from build123d import *

# Parameters (mm, degrees)
SKETCH2_W           = 115
SKETCH2_H           = 130
SKETCH2_R           = 4.8
BOSS_EXTRUDE1_DEPTH = 5
BOSS_EXTRUDE2_DEPTH = 115
SKETCH4_W           = 98.530736165
SKETCH4_H           = 115
CUT_EXTRUDE1_DEPTH  = 5
SKETCH5_R           = 4.8
CUT_EXTRUDE2_DEPTH  = 1
SKETCH6_R           = 4.8
CUT_EXTRUDE4_DEPTH  = 1
SKETCH7_W           = 19
SKETCH7_H           = 115
BOSS_EXTRUDE3_DEPTH = 39.811986363
SKETCH8_W           = 19
SKETCH8_H           = 115
SKETCH8_W_2         = 31.469263835
BOSS_EXTRUDE4_DEPTH = 100
CUT_EXTRUDE5_DEPTH  = 19
CUT_EXTRUDE6_DEPTH  = 31.469263835
CUT_EXTRUDE7_DEPTH  = 5
SKETCH12_W          = 5
SKETCH12_H          = 10
BOSS_EXTRUDE5_DEPTH = 100
CHAMFER1_SIZE       = 3
SKETCH13_W          = 5
SKETCH13_H          = 31
BOSS_EXTRUDE6_DEPTH = 5


with BuildPart() as part:
    # Sketch2 → Boss-Extrude1 (new body)
    with BuildSketch(Plane(origin=(0, 0, 0), x_dir=(0, 1, 0), z_dir=(0, 0, 1))):
        Rectangle(SKETCH2_W, SKETCH2_H)
        with Locations(Location((-18.09, -55.5, 0), (0, 0, 270))):
            Circle(SKETCH2_R, mode=Mode.SUBTRACT)
        with Locations(Location((18.08, -55.5, 0), (0, 0, 270))):
            Circle(SKETCH2_R, mode=Mode.SUBTRACT)
    extrude(amount=BOSS_EXTRUDE1_DEPTH)

    # Sketch3 → Boss-Extrude2 (add)
    with BuildSketch(Plane(origin=(0, 57.5, 0), x_dir=(-1, 0, 0), z_dir=(0, 1, 0))):
        Polygon((-65, 5), (-46, 5), (46, 45.27), (65, 45.27), (65, 39.811986363), (46, 39.811986363), (-33.530736165, 5), (-33.530736165, 0), (-65, 0), align=None)
    extrude(amount=-BOSS_EXTRUDE2_DEPTH)

    # Sketch4 → Cut-Extrude1 (cut)
    with BuildSketch(Plane.XY.offset(5)):
        with Locations((-15.734631917, 0)):
            Rectangle(SKETCH4_W, SKETCH4_H)
    extrude(amount=-CUT_EXTRUDE1_DEPTH, mode=Mode.SUBTRACT)

    # Sketch5 → Cut-Extrude2 (cut)
    with BuildSketch(Plane.XY.offset(5)):
        with Locations((56.5, 7.5)):
            Circle(SKETCH5_R)
        with Locations((56.5, -7.5)):
            Circle(SKETCH5_R)
    extrude(amount=-CUT_EXTRUDE2_DEPTH, mode=Mode.SUBTRACT)

    # Sketch6 → Cut-Extrude4 (cut)
    with BuildSketch(Plane.XY.offset(45.27)):
        with Locations((-55.5, 17.65)):
            Circle(SKETCH6_R)
        with Locations((-55.5, -17.65)):
            Circle(SKETCH6_R)
    extrude(amount=-CUT_EXTRUDE4_DEPTH, mode=Mode.SUBTRACT)

    # Sketch7 → Boss-Extrude3 (add)
    with BuildSketch(Plane(origin=(0, 0, 39.811986363), x_dir=(1, 0, 0), z_dir=(0, 0, -1))):
        with Locations((-55.5, 0)):
            Rectangle(SKETCH7_W, SKETCH7_H)
    extrude(amount=BOSS_EXTRUDE3_DEPTH)

    # Sketch8 → Boss-Extrude4 (add)
    with BuildSketch(Plane(origin=(0, 0, 0), x_dir=(1, 0, 0), z_dir=(0, 0, -1))):
        with Locations((-55.5, 0)):
            Rectangle(SKETCH8_W, SKETCH8_H)
        with Locations((49.265368083, 0)):
            Rectangle(SKETCH8_W_2, SKETCH8_H)
    extrude(amount=BOSS_EXTRUDE4_DEPTH)

    # Sketch9 → Cut-Extrude5 (cut)
    with BuildSketch(Plane(origin=(-65, 0, 0), x_dir=(0, -1, 0), z_dir=(-1, 0, 0))):
        with BuildLine():
            Line((-37.5, -95), (37.5, -95))
            ThreePointArc((37.5, -95), (44.571067812, -92.071067812), (47.5, -85))
            Line((47.5, -85), (47.5, 20.27))
            ThreePointArc((47.5, 20.27), (44.571067812, 27.341067812), (37.5, 30.27))
            Line((37.5, 30.27), (-37.5, 30.27))
            ThreePointArc((-37.5, 30.27), (-44.571067812, 27.341067812), (-47.5, 20.27))
            Line((-47.5, 20.27), (-47.5, -85))
            ThreePointArc((-47.5, -85), (-44.571067812, -92.071067812), (-37.5, -95))
        make_face()
    extrude(amount=-CUT_EXTRUDE5_DEPTH, mode=Mode.SUBTRACT)

    # Sketch10 → Cut-Extrude6 (cut)
    with BuildSketch(Plane.YZ.offset(65)):
        with BuildLine():
            Line((-40, -95), (40, -95))
            ThreePointArc((40, -95), (47.071067812, -92.071067812), (50, -85))
            Line((50, -85), (50, -15))
            ThreePointArc((50, -15), (47.071067812, -7.928932188), (40, -5))
            Line((40, -5), (-40, -5))
            ThreePointArc((-40, -5), (-47.071067812, -7.928932188), (-50, -15))
            Line((-50, -15), (-50, -85))
            ThreePointArc((-50, -85), (-47.071067812, -92.071067812), (-40, -95))
        make_face()
    extrude(amount=-CUT_EXTRUDE6_DEPTH, mode=Mode.SUBTRACT)

    # Sketch11 → Cut-Extrude7 (cut)
    with BuildSketch(Plane(origin=(9.233013436, 0, 21.093549445), x_dir=(0.9160841896254345, 0, -0.4009859816980028), z_dir=(0.4009859816980028, 0, 0.9160841896254345))):
        with BuildLine():
            Line((-40.292508114, 47.5), (20.134942814, 47.5))
            ThreePointArc((20.134942814, 47.5), (27.206010626, 44.571067812), (30.134942814, 37.5))
            Line((30.134942814, 37.5), (30.134942814, -37.5))
            ThreePointArc((30.134942814, -37.5), (27.206010626, -44.571067812), (20.134942814, -47.5))
            Line((20.134942814, -47.5), (-40.292508114, -47.5))
            ThreePointArc((-40.292508114, -47.5), (-47.363575926, -44.571067812), (-50.292508114, -37.5))
            Line((-50.292508114, -37.5), (-50.292508114, 37.5))
            ThreePointArc((-50.292508114, 37.5), (-47.363575926, 44.571067812), (-40.292508114, 47.5))
        make_face()
    extrude(amount=-CUT_EXTRUDE7_DEPTH, mode=Mode.SUBTRACT)

    # Sketch12 → Boss-Extrude5 (add)
    with BuildSketch(Plane.ZY.offset(65)):
        with Locations((-97.5, 52.5)):
            Rectangle(SKETCH12_W, SKETCH12_H)
        with Locations((-97.5, -52.5)):
            Rectangle(SKETCH12_W, SKETCH12_H)
    extrude(amount=-BOSS_EXTRUDE5_DEPTH)

    # Chamfer1
    chamfer1_edges = [part.edges().sort_by_distance(p)[0] for p in [
        (-46, 52.5, -95),
        (33.530736165, 52.5, -95),
        (-46, -52.5, -95),
        (33.530736165, -52.5, -95),
    ]]
    chamfer(chamfer1_edges, length=CHAMFER1_SIZE)

    # Sketch13 → Boss-Extrude6 (add)
    with BuildSketch(Plane(origin=(65, 0, 0), x_dir=(0, 0, -1), z_dir=(1, 0, 0))):
        with Locations((97.5, 42)):
            Rectangle(SKETCH13_W, SKETCH13_H)
    extrude(amount=BOSS_EXTRUDE6_DEPTH)


solid = part.part
Verification items for the finished model (mm, model axes). A direction names the side the tool comes from. Coordinates: 2 decimals unless noted, no trailing zeros. Write each loop counter-clockwise with the first axis right and the second up, starting at its lowest first coordinate (ties: lowest second). Pieces come first, ordered by that corner, then holes. Notation, with made-up numbers: M 45,-31 L 92,-31 A20 cw 92,-4 Z; hole C -19,73.25 d1. An arc over 180 degrees is marked long. Use CSV: the item, a comma, the result in double quotes.
Q1. Section check A-A, the plane z = -29. Enter the section's corners in (x, y), and give its area (3 significant figures).
Computed values:
outline,"M -65,-57.5 L -46,-57.5 L -46,-47.5 L -65,-47.5 Z; M -65,47.5 L -46,47.5 L -46,57.5 L -65,57.5 Z; M 33.53,-57.5 L 65,-57.5 L 65,-50 L 33.53,-50 Z; M 33.53,50 L 65,50 L 65,57.5 L 33.53,57.5 Z"
area,"852 mm²"
Q2. Go/stop test with flat-tipped pins: P1, Ø11, axis at x = 56.5, y = 7.5, coming from the +Z side; P2, Ø7.5, axis at x = -55.5, y = 17.65, coming from the +Z side; P3, Ø1, axis at x = 39, y = 32, coming from the +Z side. Record where each tip stops, or that it passes through.
Computed values:
P1,"z = 5"
P2,"z = 44.27"
P3,"z = 8.28"
Q3. Section check D-D, the plane x = -23.5. Enter the section's corners in (y, z).
Computed values:
outline,"M -57.5,-100 L -47.5,-100 L -47.5,-95 L -57.5,-95 Z; M -57.5,29.96 L -47.5,29.96 L -47.5,35.42 L -57.5,35.42 Z; M 47.5,-100 L 57.5,-100 L 57.5,-95 L 47.5,-95 Z; M 47.5,29.96 L 57.5,29.96 L 57.5,35.42 L 47.5,35.42 Z"
Q4. Set-up check for faces 1 (the flat face through (-56, 47.5, -32)), 2 (the cylindrical face through (-55.63, -44.49, -92.15)), 3 (the flat face through (-56, 18, 44.27)), 4 (the cylindrical face through (49.49, -47.15, -91.99)): record each of +Z, -Z, +X, -X, +Y, -Y from which the full face is reachable in a straight line by a thin tool's end or side.
Computed values:
face 1,"-X"
face 2,"+X, -X"
face 3,"+Z"
face 4,"+X"
Q5. Section check B-B, the plane y = -7.5. Enter the section's corners in (x, z), and give its area (3 significant figures).
Computed values:
outline,"M -65,-100 L -46,-100 L -46,-95 L -65,-95 Z; M -65,30.27 L -46,30.27 L -46,39.81 L -38.84,36.68 L -36.84,41.26 L -46,45.27 L -65,45.27 Z; M 33.53,-100 L 65,-100 L 65,-95 L 33.53,-95 Z; M 33.53,-5 L 65,-5 L 65,5 L 61.3,5 L 61.3,4 L 51.7,4 L 51.7,5 L 46,5 L 36.84,9.01 L 34.83,4.43 L 33.53,5 Z"
area,"908 mm²"
Q6. Mould release check, pull along X, two halves, no side actions. Record for faces 5 (the flat face through (-7, 52, -95)), 6 (the flat face through (70, 42, -97)), 7 (the flat face through (37, 57.5, -32)): pulls with the +X half, pulls with the -X half, needs draft (parallel to the pull), parting line crosses it, or undercut.
Computed values:
face 5,"undercut"
face 6,"pulls with the +X half"
face 7,"needs draft"
Q7. Thickness scan on line 1 along Y through (x, z) = (56.5, 4.3); line 2 along Y through (x, z) = (-55.5, 44.7); line 3 along X through (y, z) = (-48.5, -7). Record the ranges inside material, lowest first. Write a range as [from, to].
Computed values:
line 1,"[-57.5, -12.3], [-2.7, 2.7], [12.3, 57.5]"
line 2,"[-57.5, -22.45], [-12.85, 12.85], [22.45, 57.5]"
line 3,"[-65, -46], [33.53, 65]"
Q8. Section check C-C, the plane x = 56.5. Enter the section's corners in (y, z).
Computed values:
outline,"M -57.5,-100 L 57.5,-100 L 57.5,5 L 12.3,5 L 12.3,4 L 2.7,4 L 2.7,5 L -2.7,5 L -2.7,4 L -12.3,4 L -12.3,5 L -57.5,5 Z; hole M -50,-85 A10 ccw -40,-95 L 40,-95 A10 ccw 50,-85 L 50,-15 A10 ccw 40,-5 L -40,-5 A10 ccw -50,-15 Z"
